Model file for the job. Use its own axes, mm. Face numbers are marked on the shaded views. Round coordinates to 2 decimals unless told otherwise and drop trailing zeros. Order: outer loops, then holes, each group sorted by start corner. A loop starts at its lowest first (then second) coordinate and runs counter-clockwise, first axis right, second up. Notation, with made-up numbers: (67.5, -18.5) -> (113.5, -18.5) arc R28 ccw to (113.5, 0.5) -> close; hole circle Ø8 at (23.5, -9). An arc over 180 degrees is marked (long way). Answer as CSV lines item,"result".
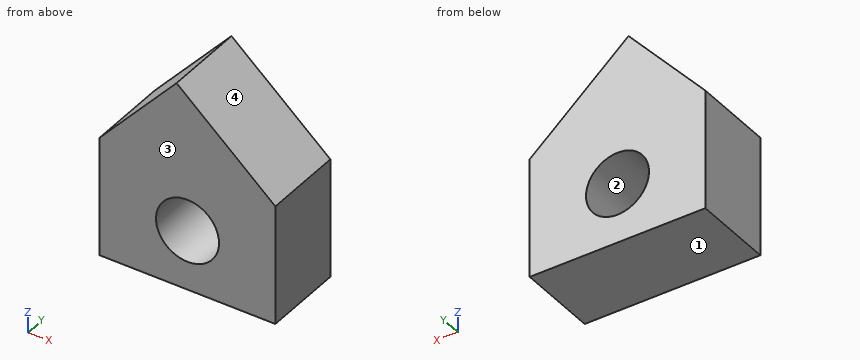
```python
from build123d import *

# Parameters (mm, degrees)
F0_W     = 54.863999
F0_H     = 37.338002
F0_R     = 9.841681
F1_DEPTH = 25.4


with BuildPart() as f1:
    # F0 (on Front) → F1 (new body)
    with BuildSketch(Plane.XZ):
        Polygon((-60.578999, 34.290002), (-5.715, 34.290002), (-36.575999, 61.150502), align=None)
        with Locations((-33.146999, 15.621001)):
            Rectangle(F0_W, F0_H)
        with Locations((-33.147, 15.621001)):
            Circle(F0_R, mode=Mode.SUBTRACT)
    extrude(amount=F1_DEPTH)


solid = f1.part
```
Q1. Saw through at B-B (z = 22). Write the cut outline in (x, y) (3 decimals), plus the area to 3 significant figures.
Checks:
outline,"(-60.579, -25.4) -> (-40.641, -25.4) -> (-40.641, 0) -> (-60.579, 0) -> close; (-25.653, -25.4) -> (-5.715, -25.4) -> (-5.715, 0) -> (-25.653, 0) -> close"
area,"1,010 mm²"
Q2. Saw through at D-D (x = -54). Write the cut outline in (y, z).
Checks:
outline,"(-25.4, -3.05) -> (0, -3.05) -> (0, 41.65) -> (-25.4, 41.65) -> close"
Q3. Saw through at A-A (x = -29.5). Write the cut outline in (y, z), plus the area to 3 significant figures.
Checks:
outline,"(-25.4, -3.05) -> (0, -3.05) -> (0, 6.48) -> (-25.4, 6.48) -> close; (-25.4, 24.76) -> (0, 24.76) -> (0, 54.99) -> (-25.4, 54.99) -> close"
area,"1,010 mm²"
Q4. Mould opens along Z. For the marked faces 1, 2, 3 and 4 say: +Z half, -Z half, draft (parallel to the pull), parting line (faces both ways), or undercut.
Checks:
face 1,"-Z half"
face 2,"undercut"
face 3,"draft"
face 4,"+Z half"
Q5. Wall check: L1, parallel to Z at x = -29.5, y = -9.5; L2, parallel to X at y = -15.5, z = 17.5 (3 decimals); L3, parallel to X at y = -20.75, z = 14.5 (3 decimals). Give the ranges that are in metal, low to high. Write a range as [from, to].
Checks:
L1,"[-3.05, 6.48], [24.76, 54.99]"
L2,"[-60.579, -42.808], [-23.486, -5.715]"
L3,"[-60.579, -42.925], [-23.369, -5.715]"
Q6. Flat gauge pin, fed straight in: pin 1 (1.5 mm diameter, centred on x = -14, y = -14.5, fed in from +Z). Where does the tip first touch, or does it go through?
Checks:
pin 1,"z = 42.15"
Q7. Saw through at C-C (y = -10). Write the cut outline in (x, z) (1 decimal).
Checks:
outline,"(-60.6, -3) -> (-5.7, -3) -> (-5.7, 34.3) -> (-36.6, 61.2) -> (-60.6, 34.3) -> close; hole circle Ø19.7 at (-33.1, 15.6)"
